Here's how the part is built. I have some questions about the finished solid (model axes, mm). Give positions to 0.01 mm unless a question says otherwise; leave off trailing zeros. Order: outer loops, then holes, each group sorted by start corner. A loop starts at its lowest first (then second) coordinate and runs counter-clockwise, first axis right, second up. Notation, with made-up numbers: (-31.5, 7) -> (-18.5, 7) arc R29 cw to (-18.5, 30) -> close; hole circle Ø7 at (-36.75, 20.25). An arc over 180 degrees is marked (long way). Write each question's results on one line, items separated by ' | '. Start each with the question number.
Q1. I'm going to push a flat-ended pin straight in: pin 1 (3 mm diameter, centred on y = 161.5, z = 13.5, fed in from +X). Where does the tip first touch, or does it pass through?
Q2. I need wall thicknesses on line 1 along Y through (x, z) = (342.5, 15.75); line 2 along Y through (x, z) = (6, 15.25); line 3 along X through (y, z) = (106, 1.5). Which ranges of each line are inside material? Lowest first, please. Write a range as [from, to].
Q3. Imagine slicing it at A-A, the plane z = 9. Please give me the cut outline in (x, y), then the cut area to 3 significant figures.
Autodesk Inventor part; units mm, degrees
ref_plane "YZ Plane" through (0, 0, 0) normal (1, 0, 0) x (0, 1, 0)
ref_plane "XZ Plane" through (0, 0, 0) normal (0, 1, 0) x (-1, 0, 0)
ref_plane "XY Plane" through (0, 0, 0) normal (0, 0, 1) x (1, 0, 0)
sketch "Sketch1" plane through (0, 0, 0) normal (1, 0, 0) x (0, 1, 0)
  line L0 (0, 0) -> (200, 0)
  line L1 (200, 0) -> (200, 20)
  line L2 (200, 20) -> (0, 20)
  line L3 (0, 20) -> (0, 0)
  dimension "d0" = 200
  dimension "d1" = 20
extrude "Extrusion1" add sketch "Sketch1" along normal blind 570
sketch "Sketch2" plane through (0, 0, 0) normal (0, 0, 1) x (1, 0, 0)
  line L0 (0, 200) -> (0, 0)
  line L1 (570, 200) -> (570, 0)
  line L2 (-90, 110) -> (-90, 0)
  line L3 (-90, 0) -> (0, 0)
  line L4 (0, 200) -> (0, 0)
  line L5 (570, 0) -> (570, 200)
  line L6 (660, 110) -> (660, 0)
  line L7 (660, 0) -> (570, 0)
  arc A0 (0, 200) -> (-90, 110) centre (0, 110) ccw
  arc A1 (660, 110) -> (570, 200) centre (570, 110) ccw
  point P0 (-40.5768, 141.5092)
  point P1 (615, 155)
  dimension "d11" = 90
  dimension "d12" = 90
extrude "Extrusion2" add sketch "Sketch2" along normal blind 20
fillet "Fillet1" radius 5 13 edges at (-90, 55, 20) (-63.6396, 173.6396, 20) (285, 200, 20) (633.6396, 173.6396, 0) (570, 200, 10) (660, 55, 0) (660, 110, 10) (-63.6396, 173.6396, 0) (0, 200, 10) (-90, 55, 0) (-90, 110, 10) (285, 200, 0) (660, 55, 20)
properties part number "Centre Wedge"
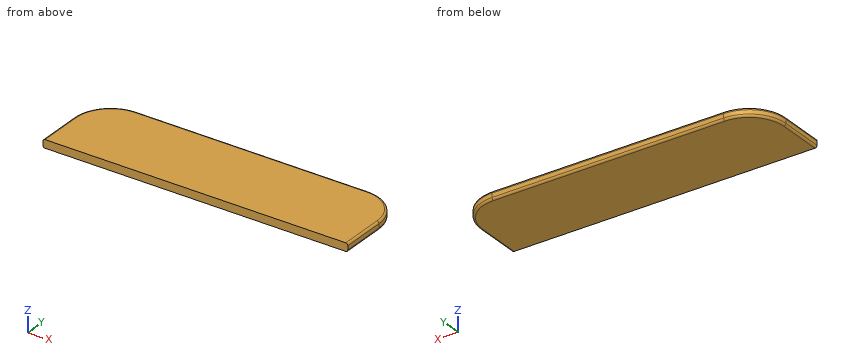
Geometry check:
1) pin 1: x = 644.83
2) line 1: [0, 199.94] | line 2: [0, 199.99] | line 3: [-88.57, 658.57]
3) outline: (-90, 0) -> (660, 0) -> (660, 110) arc R90 ccw to (570, 200) -> (0, 200) arc R90 ccw to (-90, 110) -> close | area: 147,000 mm²
